from build123d import *

# Parameters (mm, degrees)
SKETCH2_R             = 30
SKETCH2_R_2           = 27
BOSS_EXTRUDE1_DEPTH   = 10
SKETCH2_R_3           = 5
SKETCH2_R_4           = 4.5
BOSS_EXTRUDE1_2_DEPTH = 10
BOSS_EXTRUDE2_START   = -9
SKETCH4_W             = 5
SKETCH4_H             = 2
BOSS_EXTRUDE2_DEPTH   = 22.417424
CIRPATTERN1_COUNT     = 8


with BuildPart() as part:
    # Sketch2 → Boss-Extrude1 (new body)
    with BuildSketch(Plane.XY):
        Circle(SKETCH2_R)
        Circle(SKETCH2_R_2, mode=Mode.SUBTRACT)
    extrude(amount=BOSS_EXTRUDE1_DEPTH)



with BuildPart() as body_2:
    # Sketch2 → Boss-Extrude1 2 (new body)
    with BuildSketch(Plane.XY):
        Circle(SKETCH2_R_3)
        Circle(SKETCH2_R_4, mode=Mode.SUBTRACT)
    extrude(amount=BOSS_EXTRUDE1_2_DEPTH)


with BuildPart() as part_1:
    add(part.part)

    add(body_2.part)  # Boss-Extrude2 merges body 2
    # Sketch4 → Boss-Extrude2 (add)
    with BuildSketch(Plane(origin=(-18, 0, 0), x_dir=(0, 0, -1), z_dir=(1, 0, 0)).offset(BOSS_EXTRUDE2_START)):
        with Locations((-5.5, -1)):
            Rectangle(SKETCH4_W, SKETCH4_H)
    boss_extrude2 = extrude(amount=BOSS_EXTRUDE2_DEPTH)

    # CirPattern1: Boss-Extrude2 ×8 about axis
    cirpattern1_axis = Axis((0, 0, 0), (0, 0, 1))
    for i in range(1, CIRPATTERN1_COUNT):
        add(boss_extrude2.rotate(cirpattern1_axis, i * 360 / CIRPATTERN1_COUNT))


solid = part_1.part
Source: CAD feature listing. Evaluate the final solid. Frame: model axes, mm. A direction names the side the tool comes from. Give positions to 0.01 mm unless a question says otherwise; leave off trailing zeros. Order: outer loops, then holes, each group sorted by start corner. A loop starts at its lowest first (then second) coordinate and runs counter-clockwise, first axis right, second up. Notation, with made-up numbers: (-13, 36.5) -> (-5, 36.5) arc R17 cw to (-5, 67.5) -> close; hole circle Ø2 at (44, 87.25). An arc over 180 degrees is marked (long way). Write item = value, one per line.
Q1. Cut plane C-C, the plane z = 7.25. State how many separate pieces and enclosed holes the cut face has, and give its area (3 significant figures).
Data:
separate_pieces = 1
enclosed_holes = 9
area = 906 mm^2
Q2. Pin query (flat end, axial travel): pin 1 (18.5 mm diameter, centred on x = -10.5, y = 10.5, fed in from +Z); pin 2 (1.6 mm diameter, centred on x = 14, y = 0.5, fed in from -Z); pin 3 (1.5 mm diameter, centred on x = -17, z = 4.5, fed in from +Y); pin 4 (5 mm diameter, centred on x = 10.5, y = 19.5, fed in from -Z). Return the tip coordinate at first contact, or that it passes through.
Data:
pin_1 = 8
pin_2 = 3
pin_3 = 25.22
pin_4 = through
Q3. Cut plane A-A, the plane x = -24. Output: boundary loops of the cut face in (y, z), and give its area (3 significant figures).
Data:
outline = (-18, 0) -> (-12.37, 0) -> (-12.37, 10) -> (-18, 10) -> close; (-2, 3) -> (0, 3) -> (0, 8) -> (-2, 8) -> close; (12.37, 0) -> (18, 0) -> (18, 10) -> (12.37, 10) -> close
area = 123 mm^2
Q4. Pull-direction query (X, two-part tool) for faces 1 (the face through (-25, 11, 0)), 2 (the face through (-29.97, 1.32, 4.93)), 3 (the face through (2, -16, 6)); classes: released by +X, released by -X, zero draft, split by the parting line, or undercut.
Data:
face_1 = zero draft
face_2 = split by the parting line
face_3 = undercut
Q5. Cut plane D-D, the plane y = -23.5. Output: boundary loops of the cut face in (x, z).
Data:
outline = (-18.65, 0) -> (-13.29, 0) -> (-13.29, 10) -> (-18.65, 10) -> close; (0, 3) -> (2, 3) -> (2, 8) -> (0, 8) -> close; (13.29, 0) -> (18.65, 0) -> (18.65, 10) -> (13.29, 10) -> close
Q6. Cut plane B-B, the plane y = 11.5. Output: boundary loops of the cut face in (x, z).
Data:
outline = (-27.71, 0) -> (-24.43, 0) -> (-24.43, 10) -> (-27.71, 10) -> close; (-14.33, 3) -> (-11.5, 3) -> (-11.5, 8) -> (-14.33, 8) -> close; (-2, 3) -> (0, 3) -> (0, 8) -> (-2, 8) -> close; (8.67, 3) -> (11.5, 3) -> (11.5, 8) -> (8.67, 8) -> close; (24.43, 0) -> (27.71, 0) -> (27.71, 10) -> (24.43, 10) -> close
Q7. Set-up query: faces 4 (the face through (11, 11, 6)), 5 (the face through (11, 12, 8)), 6 (the face through (-12, 11, 3)), 7 (the face through (-1.08, -4.88, 4.93)). Return all of +Z, -Z, +X, -X, +Y, -Y with unobstructed straight access to the full face (end or side cutting, diameter ignored); none if empty.
Data:
face_4 = +Z, -Z
face_5 = +Z
face_6 = -Z
face_7 = none
Q8. Material intervals for line 1 (Y direction, x = 0, z = 2.5); line 2 (Y direction, x = -4, z = 4.5); line 3 (X direction, y = -11.5, z = 7), sorted ascending. Write a range as from..to.
Data:
line_1 = -30..-27, -5..-4.5, 4.5..5, 27..30
line_2 = -29.73..-26.7, -6.83..-4, -3..-2.06, 2.06..4, 26.7..29.73
line_3 = -27.71..-24.43, -11.5..-8.67, 0..2, 11.5..14.33, 24.43..27.71
